Part model, mm, in its own coordinate system. A direction names the side the tool comes from. Coordinates: 2 decimals unless noted, no trailing zeros. Loops run counter-clockwise (first coordinate to the right, second up) from the corner with the lowest first, then second, coordinate; pieces in that order, holes last. Notation, with made-up numbers: M 21,37.5 L 71,37.5 A16 cw 71,60.5 Z; hole C 17,46.25 d10. An arc over 180 degrees is marked long. Answer as a JSON object with one key per item and string values. Group by question number.
1. Saw through at B-B on z = -1345. Write the cut outline in (x, y), then the cut area to 3 significant figures.
2. Drill centre lines: L1, parallel to Z at x = -23, y = 33; L2, parallel to X at y = 24.5, z = -1460.5; L3, parallel to Z at x = -60, y = 32. Where is each one in solid material? Low to high.
3. Drop flat-ended pins along their axis: pin 1 Ø11.5 at (y, z) = (21, -150.5) entering from -X; pin 2 Ø11.5 at (x, y) = (-52, 23) entering from -Z. Give the stop position or say it passes through.
4. Saw through at A-A on y = 20. Write the cut outline in (x, z), then the cut area to 3 significant figures.
5. 3-axis set-ups, long thin cutter, end or side, ignore diameter. For faces 1 (the face through (152.4, 19, -803)), 2 (the face through (-48, 19, -451.75)), 3 (the face through (-49, 19, -1131.75)): which of +Z, -Z, +X, -X, +Y, -Y reach the whole face in a straight line?
from build123d import *

# Parameters (mm, degrees)
BOSS_EXTRUDE1_DEPTH = 38.1


with BuildPart() as part:
    # Sketch1 → Boss-Extrude1 (new body)
    with BuildSketch(Plane(origin=(0, 0, 0), x_dir=(1, 0, 0), z_dir=(0, 1, 0))):
        with BuildLine():
            Line((0, 1156.75), (0, 1583.5))
            Line((0, 1583.5), (152.4, 1583.5))
            Line((152.4, 1583.5), (152.4, 0))
            Line((152.4, 0), (0, 0))
            Line((0, 0), (0, 426.75))
            ThreePointArc((0, 426.75), (-7.32233047, 444.42766953), (-25, 451.75))
            Line((-25, 451.75), (-72.6, 451.75))
            ThreePointArc((-72.6, 451.75), (-90.27766953, 459.07233047), (-97.6, 476.75))
            Line((-97.6, 476.75), (-97.6, 1106.75))
            ThreePointArc((-97.6, 1106.75), (-90.27766953, 1124.42766953), (-72.6, 1131.75))
            Line((-72.6, 1131.75), (-25, 1131.75))
            ThreePointArc((-25, 1131.75), (-7.32233047, 1139.07233047), (0, 1156.75))
        make_face()
    extrude(amount=BOSS_EXTRUDE1_DEPTH)


solid = part.part
Outcome:
{
 "1": {"outline": "M 0,0 L 152.4,0 L 152.4,38.1 L 0,38.1 Z", "area": "5,810 mm²"},
 "2": {"L1": "z = -1131.83 to -451.67", "L2": "x = 0 to 152.4", "L3": "z = -1131.75 to -451.75"},
 "3": {"pin 1": "stops at x = 0", "pin 2": "stops at z = -1131.75"},
 "4": {"outline": "M -97.6,-1106.75 A25 ccw -72.6,-1131.75 L -25,-1131.75 A25 cw 0,-1156.75 L 0,-1583.5 L 152.4,-1583.5 L 152.4,0 L 0,0 L 0,-426.75 A25 cw -25,-451.75 L -72.6,-451.75 A25 ccw -97.6,-476.75 Z", "area": "308,000 mm²"},
 "5": {"face 1": "+Z, -Z, +X, +Y, -Y", "face 2": "+Z, -X, +Y, -Y", "face 3": "-Z, -X, +Y, -Y"}
}
